For this review, use the dimensioned drawing (mm, ordinates from the lowest corner) and the shaded views. A direction names the side the tool comes from. Give positions to 0.01 mm unless a question says otherwise; leave off trailing zeros. Order: outer loops, then holes, each group sorted by start corner. A loop starts at its lowest first (then second) coordinate and runs counter-clockwise, first axis right, second up. Notation, with made-up numbers: M 60,13.25 L 84,13.25 A34 ccw 84,52.25 Z; hole C 71.25,-32 d3. An arc over 180 degrees is marked long. One line per question, with ' | ' between items. Start each with the question number.
1. The part is to be moulded in two halves that separate along Y. For the marked faces 1, 2 and 3, say which applies: +Y half, -Y half, draft (parallel to the pull), parting line (faces both ways), or undercut.
2. We need section C-C on y = 8. Write out the cut boundary in (x, z).
3. We need section B-B on z = 4.5. Write out the cut boundary in (x, y).
4. Insertion check: P1, Ø1, axis at x = 6, z = 5, coming from the +Y side; P2, Ø1.5, axis at x = 2, z = 1.5, coming from the +Y side (1 decimal); P3, Ø1.5, axis at x = 7, y = 7, coming from the +Z side; P4, Ø4, axis at x = 3, y = 8.5, coming from the +Z side. Each pin has a flat end and moves straight along its axis. Give the tip position at first contact, or say it passes through.
5. We need section D-D on x = 1.5. Write out the cut boundary in (y, z).
6. We need section A-A on z = 1.25. Write out the cut boundary in (x, y).
7. For the marked faces 4, 5 and 6, list the 3-axis set-ups (+Z, -Z, +X, -X, +Y, -Y) from which the entire face can be reached by the end or side of a thin tool; tool diameter is ignored.
8. Wall thickness on L1, parallel to Z at x = 2.5, y = 5.75; L2, parallel to Z at x = 2, y = 1.5; L3, parallel to Y at x = 3.25, z = 5.75: over which ranges is each line inside the solid? List them lowest first.
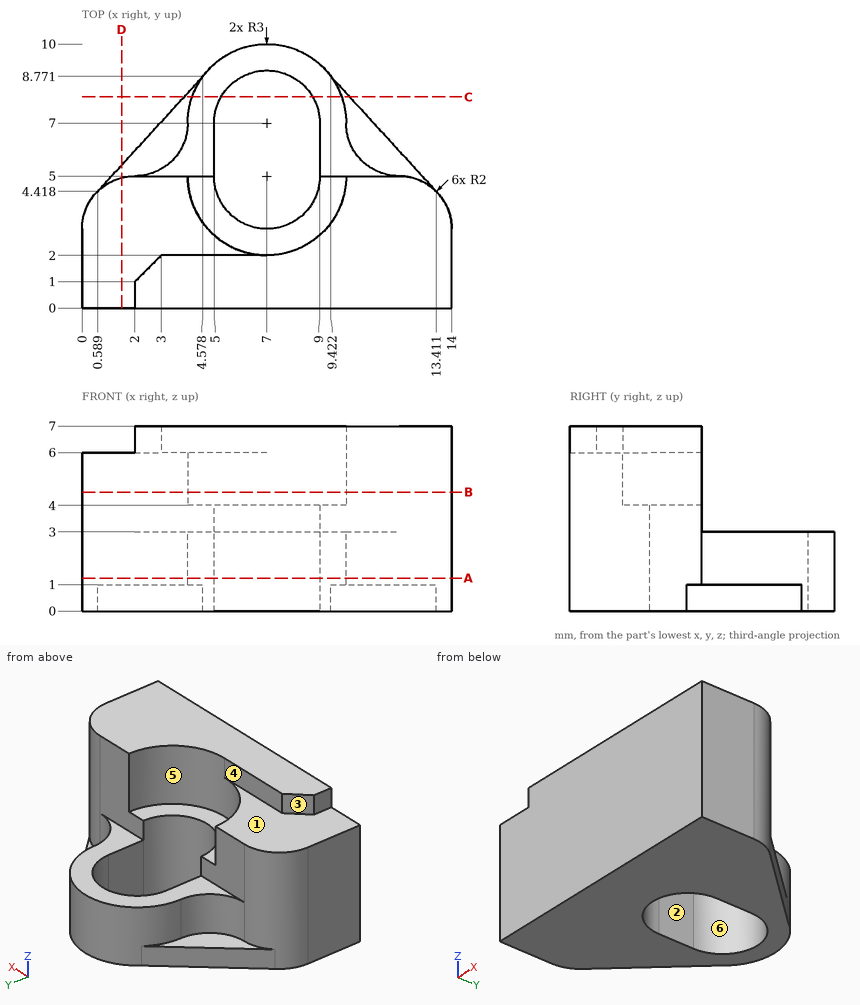
Entries:
1) face 1: draft | face 2: undercut | face 3: +Y half
2) outline: M 3.87,0 L 5.27,0 L 5.27,3 L 4.17,3 L 4.17,1 L 3.87,1 Z; M 8.73,0 L 10.13,0 L 10.13,1 L 9.83,1 L 9.83,3 L 8.73,3 Z
3) outline: M 0,0 L 14,0 L 14,3 A2 ccw 12,5 L 10,5 A3 cw 4,5 L 2,5 A2 ccw 0,3 Z
4) P1: stops at y = 2.4 | P2: stops at y = 6.6 | P3: passes through | P4: stops at z = 3
5) outline: M 0,0 L 5.41,0 L 5.41,1 L 4.94,1 L 4.94,6 L 0,6 Z
6) outline: M 0,0 L 14,0 L 14,3 A2 ccw 12,5 A2 cw 10,7 A3 ccw 4,7 A2 cw 2,5 A2 ccw 0,3 Z; hole M 5,5 A2 ccw 9,5 L 9,7 A2 ccw 5,7 Z
7) face 4: +Z, -X, +Y | face 5: +Z, +Y | face 6: +Z, -Z
8) L1: z = 0 to 1 | L2: z = 0 to 6 | L3: y = 0 to 5
